Read the model definition and answer for the solid it produces. Units are mm, in the model's axes. Round coordinates to 2 decimals unless told otherwise and drop trailing zeros. Write each loop counter-clockwise with the first axis right and the second up, starting at its lowest first coordinate (ties: lowest second). Pieces come first, ordered by that corner, then holes. Notation, with made-up numbers: (72.5, 60) - (101.5, 60) arc R15 cw to (101.5, 88) - close; hole circle Ø3 at (-6.5, 65). An arc over 180 degrees is marked (long way). Answer as CSV lines item,"result". Start each with the question number.
1) Find section A-A on x = 54. Determine the outline of the cut face in (y, z).
2) Consider line 1 along Y through (x, z) = (70.5, 0.9); line 2 along Y through (x, z) = (106.5, 0.3); line 3 along X through (y, z) = (18.75, 0.25). Determine where each line is inside the solid, lowest interval first.
3) Find section C-C on x = 106.5. Determine the outline of the cut face in (y, z).
4) Find section D-D on y = 31. Determine the outline of the cut face in (x, z), then the cut area to 3 significant figures.
5) Find section B-B on y = 18.75. Determine the outline of the cut face in (x, z), then the cut area to 3 significant figures.
Autodesk Inventor part; units mm, degrees
ref_plane "YZ Plane" through (0, 0, 0) normal (1, 0, 0) x (0, 1, 0)
ref_plane "XZ Plane" through (0, 0, 0) normal (0, 1, 0) x (-1, 0, 0)
ref_plane "XY Plane" through (0, 0, 0) normal (0, 0, 1) x (1, 0, 0)
sketch "Skizze1" plane through (0, 0, 0) normal (0, 0, 1) x (1, 0, 0)
  line L0 (0, 0) -> (127, 0)
  line L1 (127, 0) -> (127, 37.5)
  line L2 (127, 37.5) -> (0, 37.5)
  line L3 (0, 37.5) -> (0, 0)
  line L4 (4.75, 3.65) -> (14.75, 3.65)
  line L5 (14.75, 3.65) -> (14.75, 13.85)
  line L6 (14.75, 13.85) -> (4.75, 13.85)
  line L7 (4.75, 13.85) -> (4.75, 3.65)
  line L8 (4.75, 33.85) -> (4.75, 23.65)
  line L9 (14.75, 33.85) -> (4.75, 33.85)
  line L10 (14.75, 23.65) -> (14.75, 33.85)
  line L11 (4.75, 23.65) -> (14.75, 23.65)
  line L12 (26.25, 13.85) -> (26.25, 3.65)
  line L13 (36.25, 13.85) -> (26.25, 13.85)
  line L14 (36.25, 3.65) -> (36.25, 13.85)
  line L15 (26.25, 3.65) -> (36.25, 3.65)
  line L16 (26.25, 33.85) -> (26.25, 23.65)
  line L17 (36.25, 33.85) -> (26.25, 33.85)
  line L18 (36.25, 23.65) -> (36.25, 33.85)
  line L19 (26.25, 23.65) -> (36.25, 23.65)
  line L20 (47.75, 13.85) -> (47.75, 3.65)
  line L21 (57.75, 13.85) -> (47.75, 13.85)
  line L22 (57.75, 3.65) -> (57.75, 13.85)
  line L23 (47.75, 3.65) -> (57.75, 3.65)
  line L24 (47.75, 33.85) -> (47.75, 23.65)
  line L25 (57.75, 33.85) -> (47.75, 33.85)
  line L26 (57.75, 23.65) -> (57.75, 33.85)
  line L27 (47.75, 23.65) -> (57.75, 23.65)
  line L28 (69.25, 13.85) -> (69.25, 3.65)
  line L29 (79.25, 13.85) -> (69.25, 13.85)
  line L30 (79.25, 3.65) -> (79.25, 13.85)
  line L31 (69.25, 3.65) -> (79.25, 3.65)
  line L32 (69.25, 33.85) -> (69.25, 23.65)
  line L33 (79.25, 33.85) -> (69.25, 33.85)
  line L34 (79.25, 23.65) -> (79.25, 33.85)
  line L35 (69.25, 23.65) -> (79.25, 23.65)
  line L36 (90.75, 13.85) -> (90.75, 3.65)
  line L37 (100.75, 13.85) -> (90.75, 13.85)
  line L38 (100.75, 3.65) -> (100.75, 13.85)
  line L39 (90.75, 3.65) -> (100.75, 3.65)
  line L40 (90.75, 33.85) -> (90.75, 23.65)
  line L41 (100.75, 33.85) -> (90.75, 33.85)
  line L42 (100.75, 23.65) -> (100.75, 33.85)
  line L43 (90.75, 23.65) -> (100.75, 23.65)
  line L44 (112.25, 13.85) -> (112.25, 3.65)
  line L45 (122.25, 13.85) -> (112.25, 13.85)
  line L46 (122.25, 3.65) -> (122.25, 13.85)
  line L47 (112.25, 3.65) -> (122.25, 3.65)
  line L48 (112.25, 33.85) -> (112.25, 23.65)
  line L49 (122.25, 33.85) -> (112.25, 33.85)
  line L50 (122.25, 23.65) -> (122.25, 33.85)
  line L51 (112.25, 23.65) -> (122.25, 23.65)
  arc A0 (109.2272, 0) -> (103.7728, 0) centre (106.5, -1.25) ccw
  arc A1 (103.7728, 37.5) -> (109.2272, 37.5) centre (106.5, 38.75) ccw
  point P0 (0, 18.75)
  point P1 (63.5, 37.5)
  point P2 (42, 18.75)
  point P3 (85, 18.75)
  point P4 (63.5, 0)
  point P5 (4.75, 28.75)
  point P6 (95.75, 3.65)
  point P7 (106.5, 18.75)
  dimension "d0" = 127
  dimension "d1" = 37.5
  dimension "d2" = 10.2
  dimension "d3" = 10
  dimension "d6" = 20
  dimension "d9" = 21.5
  dimension "d13" = 5.75
  dimension "d17" = 43
  dimension "d18" = 21.5
  dimension "d19" = 10
  dimension "d20" = 3
  dimension "d21" = 1.25
  dimension "d22" = 10.75
  dimension "d23" = 1.25
extrude "Extrusion1" add sketch "Skizze1" along normal blind 1 contours L3 L2 A1 L1 L0 A0
fillet "Rundung1" radius 5 4 edges at (127, 37.5, 0.5) (127, 0, 0.5) (0, 37.5, 0.5) (0, 0, 0.5)
fillet "Rundung2" radius 3 4 edges at (103.7728, 0, 0.5) (109.2272, 0, 0.5) (103.7728, 37.5, 0.5) (109.2272, 37.5, 0.5)
hole "Bohrung1" at (106.5, 18.75, 0) direction (0, 0, 1) diameter 5 end through all
sketch "Skizze2" plane through (0, 0, 1) normal (0, 0, 1) x (1, 0, 0)
  arc A0 (0, 5) -> (5, 0) centre (5, 5) ccw
  line L0 (5, 0) -> (102.2647, 0)
  arc A1 (122, 0) -> (127, 5) centre (122, 5) ccw
  line L1 (127, 5) -> (127, 32.5)
  arc A2 (127, 32.5) -> (122, 37.5) centre (122, 32.5) ccw
  line L2 (122, 37.5) -> (110.7353, 37.5)
  arc A3 (5, 37.5) -> (0, 32.5) centre (5, 32.5) ccw
  line L3 (0, 32.5) -> (0, 5)
  line L4 (112.25, 33.85) -> (122.25, 33.85)
  line L5 (122.25, 33.85) -> (122.25, 23.65)
  line L6 (122.25, 23.65) -> (112.25, 23.65)
  line L7 (112.25, 23.65) -> (112.25, 33.85)
  line L8 (112.25, 13.85) -> (122.25, 13.85)
  line L9 (122.25, 13.85) -> (122.25, 3.65)
  line L10 (122.25, 3.65) -> (112.25, 3.65)
  line L11 (112.25, 3.65) -> (112.25, 13.85)
  line L12 (90.75, 33.85) -> (100.75, 33.85)
  line L13 (100.75, 33.85) -> (100.75, 23.65)
  line L14 (100.75, 23.65) -> (90.75, 23.65)
  line L15 (90.75, 23.65) -> (90.75, 33.85)
  line L16 (90.75, 13.85) -> (100.75, 13.85)
  line L17 (100.75, 13.85) -> (100.75, 3.65)
  line L18 (100.75, 3.65) -> (90.75, 3.65)
  line L19 (90.75, 3.65) -> (90.75, 13.85)
  line L20 (69.25, 33.85) -> (79.25, 33.85)
  line L21 (79.25, 33.85) -> (79.25, 23.65)
  line L22 (79.25, 23.65) -> (69.25, 23.65)
  line L23 (69.25, 23.65) -> (69.25, 33.85)
  line L24 (69.25, 13.85) -> (79.25, 13.85)
  line L25 (79.25, 13.85) -> (79.25, 3.65)
  line L26 (79.25, 3.65) -> (69.25, 3.65)
  line L27 (69.25, 3.65) -> (69.25, 13.85)
  line L28 (47.75, 33.85) -> (57.75, 33.85)
  line L29 (57.75, 33.85) -> (57.75, 23.65)
  line L30 (57.75, 23.65) -> (47.75, 23.65)
  line L31 (47.75, 23.65) -> (47.75, 33.85)
  line L32 (47.75, 13.85) -> (57.75, 13.85)
  line L33 (57.75, 13.85) -> (57.75, 3.65)
  line L34 (57.75, 3.65) -> (47.75, 3.65)
  line L35 (47.75, 3.65) -> (47.75, 13.85)
  line L36 (26.25, 33.85) -> (36.25, 33.85)
  line L37 (36.25, 33.85) -> (36.25, 23.65)
  line L38 (36.25, 23.65) -> (26.25, 23.65)
  line L39 (26.25, 23.65) -> (26.25, 33.85)
  line L40 (26.25, 13.85) -> (36.25, 13.85)
  line L41 (36.25, 13.85) -> (36.25, 3.65)
  line L42 (36.25, 3.65) -> (26.25, 3.65)
  line L43 (26.25, 3.65) -> (26.25, 13.85)
  line L44 (4.75, 33.85) -> (14.75, 33.85)
  line L45 (14.75, 33.85) -> (14.75, 23.65)
  line L46 (14.75, 23.65) -> (4.75, 23.65)
  line L47 (4.75, 23.65) -> (4.75, 33.85)
  line L48 (4.75, 3.65) -> (4.75, 13.85)
  line L49 (4.75, 13.85) -> (14.75, 13.85)
  line L50 (14.75, 13.85) -> (14.75, 3.65)
  line L51 (14.75, 3.65) -> (4.75, 3.65)
  arc A4 (108.6176, 0.875) -> (104.3824, 0.875) centre (106.5, -1.25) ccw
  line L52 (110.7353, 0) -> (122, 0)
  arc A5 (104.3824, 36.625) -> (108.6176, 36.625) centre (106.5, 38.75) ccw
  line L53 (102.2647, 37.5) -> (5, 37.5)
  arc A6 (110.7353, 37.5) -> (108.6176, 36.625) centre (110.7353, 34.5) ccw
  arc A7 (104.3824, 36.625) -> (102.2647, 37.5) centre (102.2647, 34.5) ccw
  arc A8 (102.2647, 0) -> (104.3824, 0.875) centre (102.2647, 3) ccw
  arc A9 (108.6176, 0.875) -> (110.7353, 0) centre (110.7353, 3) ccw
  point P0 (0, 0)
equation "\"d23\" = d21"
equation "\"Biegeradius\" = Stärke"
equation "\"BreiteBiegungsfreistellung\" = Stärke"
equation "\"TiefeBiegungsfreistellung\" = 0.5 * Stärke"
equation "\"GrößeEckenfreistellung\" = 4 * Stärke"
equation "\"MinimalRest\" = 2 * Stärke"
equation "\"Übergangsradius\" = Biegeradius"
equation "\"JacobiRadiusGröße\" = Biegeradius"
equation "\"Abstandsgröße\" = Stärke"
properties part number "bat_contacts_v2_plate" material "Kupfer"
Check values:
1,outline,"(0, 0) - (3.65, 0) - (3.65, 1) - (0, 1) - close; (13.85, 0) - (23.65, 0) - (23.65, 1) - (13.85, 1) - close; (33.85, 0) - (37.5, 0) - (37.5, 1) - (33.85, 1) - close"
2,line 1,"y = 0 to 3.65, 13.85 to 23.65, 33.85 to 37.5"
2,line 2,"y = 1.75 to 16.25, 21.25 to 35.75"
2,line 3,"x = 0 to 104, 109 to 127"
3,outline,"(1.75, 0) - (16.25, 0) - (16.25, 1) - (1.75, 1) - close; (21.25, 0) - (35.75, 0) - (35.75, 1) - (21.25, 1) - close"
4,outline,"(0, 0) - (4.75, 0) - (4.75, 1) - (0, 1) - close; (14.75, 0) - (26.25, 0) - (26.25, 1) - (14.75, 1) - close; (36.25, 0) - (47.75, 0) - (47.75, 1) - (36.25, 1) - close; (57.75, 0) - (69.25, 0) - (69.25, 1) - (57.75, 1) - close; (79.25, 0) - (90.75, 0) - (90.75, 1) - (79.25, 1) - close; (100.75, 0) - (112.25, 0) - (112.25, 1) - (100.75, 1) - close; (122.25, 0) - (127, 0) - (127, 1) - (122.25, 1) - close"
4,area,"67.0 mm^2"
5,outline,"(0, 0) - (104, 0) - (104, 1) - (0, 1) - close; (109, 0) - (127, 0) - (127, 1) - (109, 1) - close"
5,area,"122 mm^2"
